Autodesk Inventor part; units mm, degrees
ref_plane "YZ Plane" through (0, 0, 0) normal (1, 0, 0) x (0, 1, 0)
ref_plane "XZ Plane" through (0, 0, 0) normal (0, 1, 0) x (-1, 0, 0)
ref_plane "XY Plane" through (0, 0, 0) normal (0, 0, 1) x (1, 0, 0)
sketch "草圖1" plane through (0, 0, 0) normal (0, 0, 1) x (1, 0, 0)
  line L0 (0, 0) -> (80, 0)
  line L1 (80, 0) -> (80, 10)
  line L2 (80, 10) -> (0, 10)
  line L3 (0, 10) -> (0, 0)
  dimension "d0" = 80
  dimension "d1" = 10
extrude "擠出1" add sketch "草圖1" along normal blind 30
sketch "草圖2" plane through (0, 0, 30) normal (0, 0, 1) x (1, 0, 0)
  line L0 (80, 10) -> (0, 10)
  line L1 (20, 10) -> (60, 10)
  line L2 (60, 10) -> (60, 40)
  line L3 (60, 40) -> (20, 40)
  line L4 (20, 40) -> (20, 10)
  point P0 (0, 0)
  dimension "d4" = 20
  dimension "d5" = 20
  dimension "d6" = 30
extrude "擠出2" add sketch "草圖2" against normal up to surface (30 mm away)
sketch "草圖3" plane through (0, 0, 30) normal (0, 0, 1) x (1, 0, 0)
  line L0 (60, 40) -> (20, 40)
  circle A0 centre (40, 40) radius 10
  point P0 (0, 0)
  dimension "d9" = 20
extrude "擠出3" cut sketch "草圖3" against normal blind 30
sketch "草圖4" plane through (0, 0, 30) normal (0, 0, 1) x (1, 0, 0)
  arc A0 (30, 40) -> (50, 40) centre (40, 40) ccw
  line L0 (30, 40) -> (20, 40)
  circle A1 centre (40, 40) radius 20
  circle A2 centre (40, 40) radius 10
  line L1 (20, 40) -> (30, 40)
  line L2 (60, 40) -> (50, 40)
  line L3 (50, 40) -> (60, 40)
  line L4 (60, 10) -> (60, 40)
  point P0 (0, 0)
extrude "擠出4" add sketch "草圖4" along normal blind 10 contours A0 L2 A1 L0
properties part number "1"
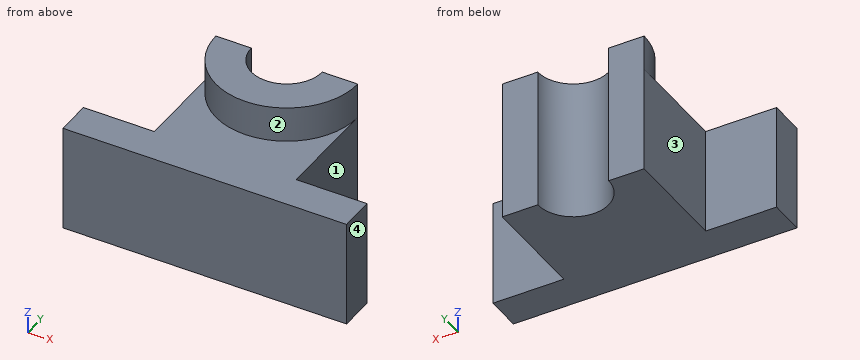
Here's how the part is built. I have some questions about the finished solid (model axes, mm). Face numbers are marked on the shaded views. A direction names the side the tool comes from. Coordinates: 2 decimals unless noted, no trailing zeros. Order: outer loops, then holes, each group sorted by start corner. A loop starts at its lowest first (then second) coordinate and runs counter-clockwise, first axis right, second up. Notation, with made-up numbers: M 38.25,-2.5 L 46.25,-2.5 A15 ccw 46.25,13.5 Z; hole C 73,59.25 d3. An arc over 180 degrees is marked long. Answer as CSV lines item,"result".
Item 1: Imagine slicing it at B-B on z = 28.5. Write out the boundary of the cut face in (x, y), plus the area to 3 significant figures.
Results found:
outline,"M 0,0 L 80,0 L 80,10 L 60,10 L 60,40 L 50,40 A10 cw 30,40 L 20,40 L 20,10 L 0,10 Z"
area,"1,840 mm2"
Item 2: On a 3-axis mill with a long thin cutter (end or side, diameter ignored), from which of +Z, -Z, +X, -X, +Y, -Y can I reach the whole of each face in a straight line? I mean the marked faces 1, 2, 3 and 4. Say none if no direction works.
Results found:
face 1,"+Z, -Z, +X, +Y"
face 2,"+Z, -Y"
face 3,"+Z, -Z, -X, +Y"
face 4,"+Z, -Z, +X, +Y, -Y"
Item 3: Imagine slicing it at D-D on x = 27. Write out the boundary of the cut face in (y, z), plus the area to 3 significant figures.
Results found:
outline,"M 0,0 L 40,0 L 40,40 L 24.8,40 L 24.8,30 L 0,30 Z"
area,"1,350 mm2"
Item 4: Imagine slicing it at A-A on x = 40. Write out the boundary of the cut face in (y, z).
Results found:
outline,"M 0,0 L 30,0 L 30,40 L 20,40 L 20,30 L 0,30 Z"
Item 5: For pin 1 (4 mm diameter, centred on x = 66, z = 26.5, fed in from +Y); pin 2 (8 mm diameter, centred on x = 52, y = 4.5, fed in from +Z); pin 3 (15 mm diameter, centred on y = 22.5, z = 11, fed in from -X); pin 4 (1 mm diameter, centred on x = 62, y = 13, fed in from -Z), each with a flat end and sliding along its axis, tell me the tip position at first contact or that it passes through.
Results found:
pin 1,"y = 10"
pin 2,"z = 30"
pin 3,"x = 20"
pin 4,"through"
Item 6: If I drill on line 1 (X direction, y = 16, z = 6.5); line 2 (Y direction, x = 72, z = 7.5); line 3 (Z direction, x = 22.5, y = 27.5), over which ranges is the centre line in solid material (lowest first)?
Results found:
line 1,"20 to 60"
line 2,"0 to 10"
line 3,"0 to 30"
Item 7: Imagine slicing it at C-C on y = 27.5. Write out the boundary of the cut face in (x, z).
Results found:
outline,"M 20,0 L 60,0 L 60,30 L 55.61,30 L 55.61,40 L 24.39,40 L 24.39,30 L 20,30 Z"
